Part model, mm, in its own coordinate system. Face numbers are marked on the shaded views. A direction names the side the tool comes from. Coordinates: 2 decimals unless noted, no trailing zeros. Order: outer loops, then holes, each group sorted by start corner. A loop starts at its lowest first (then second) coordinate and runs counter-clockwise, first axis right, second up.
1) Tool access for the marked faces 1, 2 and 3: list every direction of +Z, -Z, +X, -X, +Y, -Y with a clear straight run to the whole face (end or side of a thin tool).
2) Wall check: L1, parallel to X at y = -47, z = 87; L2, parallel to X at y = -0.5, z = 92.5; L3, parallel to Y at x = 39, z = 99.5. Give the ranges that are in metal, low to high.
3) Cut at A-A (z = 47). List the corners of the cut face in (x, y), and give its area (3 significant figures).
4) Pin check, flat tips, straight feed: pin 1 Ø2 at (y, z) = (-14, 90) entering from +X; pin 2 Ø10 at (x, z) = (25, 71) entering from +Y; pin 3 Ø9.5 at (y, z) = (-39.5, 52) entering from +X. Stop position of each tip, or through.
5) Cut at B-B (y = 20.5). List the corners of the cut face in (x, z), and give its area (3 significant figures).
6) Cut at C-C (x = 28.5). List the corners of the cut face in (y, z).
```python
from build123d import *

# Parameters (mm, degrees)
F1_DEPTH = 119.888
F2_R     = 5.08


with BuildPart() as f1:
    # F0 (on Top) → F1 (new body)
    with BuildSketch(Plane.XY):
        with BuildLine():
            Line((0, -19.529681), (0, 0))
            Line((0, 0), (74.540958, 0))
            Line((74.540958, 0), (74.540958, -28.357976))
            ThreePointArc((74.540958, -28.357976), (82.094388, -15.063883), (84.714819, 0))
            ThreePointArc((84.714819, 0), (30.085314, 43.468405), (0, -19.529681))
        make_face()
        with BuildLine():
            Line((74.540958, 0), (0, 0))
            Line((0, 0), (0, -19.529681))
            ThreePointArc((0, -19.529681), (34.859712, -44.298934), (74.540958, -28.357976))
            Line((74.540958, -28.357976), (74.540958, 0))
        make_face()
        with BuildLine():
            ThreePointArc((74.540958, -28.357976), (34.859712, -44.298934), (0, -19.529681))
            Line((0, -19.529681), (0, -52.259699))
            Line((0, -52.259699), (74.540958, -52.259699))
            Line((74.540958, -52.259699), (74.540958, -28.357976))
        make_face()
    extrude(amount=F1_DEPTH)

    # F2
    f2_edges = [f1.edges().sort_by_distance(p)[0] for p in [
        (74.540958, -52.259699, 59.944),
    ]]
    fillet(f2_edges, radius=F2_R)


solid = f1.part
```
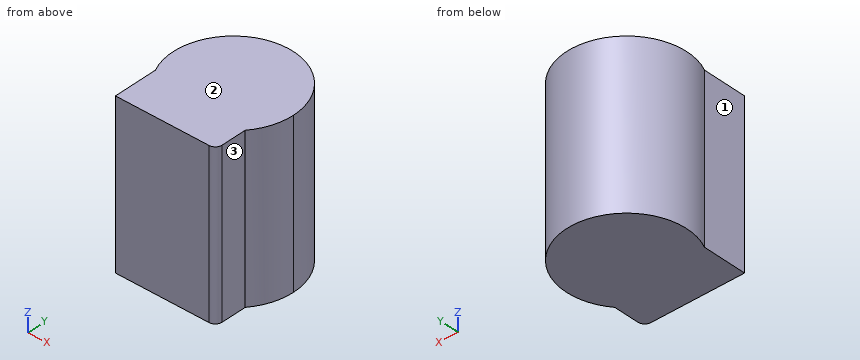
Geometry check:
1. face 1: +Z, -Z, -X, -Y
1. face 2: +Z, +X, -X, +Y, -Y
1. face 3: +Z, -Z, +X, -Y
2. L1: x = 0 to 74.54
2. L2: x = -4.5 to 84.71
2. L3: y = -52.26 to 44.59
3. outline: (0, -52.26) - (69.46, -52.26) arc R5.08 ccw to (74.54, -47.18) - (74.54, -28.36) arc R44.61 ccw to (84.71, 0) arc R44.61 ccw (long way) to (0, -19.53) - close
3. area: 7,270 mm2
4. pin 1: stops at x = 82.78
4. pin 2: stops at y = 43.45
4. pin 3: stops at x = 74.54
5. outline: (0.49, 0) - (79.73, 0) - (79.73, 119.89) - (0.49, 119.89) - close
5. area: 9,500 mm2
6. outline: (-52.26, 0) - (43.07, 0) - (43.07, 119.89) - (-52.26, 119.89) - close
